Model file for the job. Use its own axes, mm. A direction names the side the tool comes from. Round coordinates to 2 decimals unless told otherwise and drop trailing zeros. Order: outer loops, then holes, each group sorted by start corner. A loop starts at its lowest first (then second) coordinate and runs counter-clockwise, first axis right, second up. Notation, with made-up numbers: (20, 87) -> (50, 87) arc R25 cw to (50, 101) -> close; hole circle Ø6 at (-10.75, 57.5). An arc over 180 degrees is marked (long way). Put each result on its own line as item: value. Start each with the question number.
Q1. Cut at C-C, the plane x = 2. List the corners of the cut face in (y, z), and give its area (3 significant figures).
Q2. Probe L1, parallel to Z at x = 3.5, y = 2.5; L2, parallel to Y at x = 9.62, z = 1.5; L3, parallel to X at y = -2, z = -49. List the from-to ranges inside material, lowest first.
Q3. 3-axis set-ups, long thin cutter, end or side, ignore diameter. For faces 4 (the face through (-15.889, 10.106, -54.845)), 5 (the face through (-11.96, 18.73, -4.93)), 6 (the face through (-13, 0.05, -4)), 7 (the face through (9.322, 1.373, 1.217)): which of +Z, -Z, +X, -X, +Y, -Y reach the whole face in a straight line?
Q4. Flat gauge pins, fed straight in: P1, Ø6, axis at x = -12.5, z = -17.5, coming from the -Y side; P2, Ø3, axis at x = -14.5, z = -6.5, coming from the -Y side; P3, Ø2, axis at x = 9.62, y = 2.715, coming from the +Z side; P4, Ø8, axis at x = -13, z = -5.5, coming from the +Y side. Where does each tip first touch, or does it go through?
Q5. Cut at D-D, the plane x = 9.62. List the corners of the cut face in (y, z) (3 decimals), and give its area (3 significant figures).
Q6. Cut at B-B, the plane y = 10. List the corners of the cut face in (x, z) (3 decimals).
Q7. Pull direction Y, two halves, no side cores. Call faces 1 (the face through (16.726, 11.363, 1.217)), 2 (the face through (-13, 0.05, -52)), 3 (the face through (-17.889, 10.245, -57.245)): released by +Y, released by -Y, zero draft, split by the parting line, or undercut.
Q8. Cut at A-A, the plane z = -8.5. List the corners of the cut face in (x, y), and give its area (3 significant figures).
from build123d import *

# Parameters (mm, degrees)
BOSS_EXTRUDE1_DEPTH = 2.4
BOSS_EXTRUDE2_DEPTH = 2.4
SKETCH2_W           = 2
SKETCH2_H           = 35
BOSS_EXTRUDE3_DEPTH = 60.848228
CUT_EXTRUDE1_REACH  = 62.848
SKETCH4_R           = 1.575
CUT_EXTRUDE2_REACH  = 62.848
SKETCH6_R           = 3.41
SKETCH6_R_2         = 1.375
FILLET1_R           = 4
BOSS_EXTRUDE4_DEPTH = 1.2
BOSS_EXTRUDE5_DEPTH = 1.2


with BuildPart() as part:
    # Sketch1 → Boss-Extrude1 (new body)
    with BuildSketch(Plane.XY):
        with BuildLine():
            Line((12.127473017, -0.607666052), (-17.03, -7.5))
            Line((-17.03, -7.5), (-17.03, 27.5))
            Line((-17.03, 27.5), (12.127473017, 20.607666052))
            ThreePointArc((12.127473017, 20.607666052), (20.52, 10), (12.127473017, -0.607666052))
        make_face()
    extrude(amount=BOSS_EXTRUDE1_DEPTH)



with BuildPart() as body_2:
    # Sketch3 → Boss-Extrude2 (new body)
    with BuildSketch(Plane(origin=(0, 0, -56.04822809), x_dir=(-1, 0, 0), z_dir=(0, 0, -1))):
        with BuildLine():
            Line((-12.127473017, -0.607666052), (17.03, -7.5))
            Line((17.03, -7.5), (17.03, 27.5))
            Line((17.03, 27.5), (-12.127473017, 20.607666052))
            ThreePointArc((-12.127473017, 20.607666052), (-20.52, 10), (-12.127473017, -0.607666052))
        make_face()
    extrude(amount=BOSS_EXTRUDE2_DEPTH)


with BuildPart() as part_1:
    add(part.part)

    add(body_2.part)  # Boss-Extrude3 merges body 2
    # Sketch2 → Boss-Extrude3 (add)
    with BuildSketch(Plane.XY.offset(2.4)):
        with Locations((-18.03, 10)):
            Rectangle(SKETCH2_W, SKETCH2_H)
    extrude(amount=-BOSS_EXTRUDE3_DEPTH)

    # Sketch4 → Cut-Extrude1 (cut, up to next)
    with BuildSketch(Plane(origin=(0, 0, -58.44822809), x_dir=(-1, 0, 0), z_dir=(0, 0, -1)), mode=Mode.PRIVATE) as cut_extrude1_sk1:
        with Locations((-9.62, 10)):
            Circle(SKETCH4_R)
    cut_extrude1_tool1 = extrude(cut_extrude1_sk1.sketch, amount=-CUT_EXTRUDE1_REACH, mode=Mode.PRIVATE) & part_1.part
    add(cut_extrude1_tool1.solids().sort_by_distance((9.62, 10, -58.448228))[0], mode=Mode.SUBTRACT)

    # Sketch6 → Cut-Extrude2 (cut, up to next)
    with BuildSketch(Plane.XY.offset(2.4), mode=Mode.PRIVATE) as cut_extrude2_sk1:
        with Locations((9.62, 10)):
            Circle(SKETCH6_R)
    cut_extrude2_tool1 = extrude(cut_extrude2_sk1.sketch, amount=-CUT_EXTRUDE2_REACH, mode=Mode.PRIVATE) & part_1.part
    add(cut_extrude2_tool1.solids().sort_by_distance((9.62, 10, 2.4))[0], mode=Mode.SUBTRACT)
    # Sketch6 → Cut-Extrude2 (cut, up to next)
    with BuildSketch(Plane.XY.offset(2.4), mode=Mode.PRIVATE) as cut_extrude2_sk2:
        with Locations((2.335, 10)):
            Circle(SKETCH6_R_2)
    cut_extrude2_tool2 = extrude(cut_extrude2_sk2.sketch, amount=-CUT_EXTRUDE2_REACH, mode=Mode.PRIVATE) & part_1.part
    add(cut_extrude2_tool2.solids().sort_by_distance((2.335, 10, 2.4))[0], mode=Mode.SUBTRACT)
    # Sketch6 → Cut-Extrude2 (cut, up to next)
    with BuildSketch(Plane.XY.offset(2.4), mode=Mode.PRIVATE) as cut_extrude2_sk3:
        with Locations((9.62, 17.285)):
            Circle(SKETCH6_R_2)
    cut_extrude2_tool3 = extrude(cut_extrude2_sk3.sketch, amount=-CUT_EXTRUDE2_REACH, mode=Mode.PRIVATE) & part_1.part
    add(cut_extrude2_tool3.solids().sort_by_distance((9.62, 17.285, 2.4))[0], mode=Mode.SUBTRACT)
    # Sketch6 → Cut-Extrude2 (cut, up to next)
    with BuildSketch(Plane.XY.offset(2.4), mode=Mode.PRIVATE) as cut_extrude2_sk4:
        with Locations((16.905, 10)):
            Circle(SKETCH6_R_2)
    cut_extrude2_tool4 = extrude(cut_extrude2_sk4.sketch, amount=-CUT_EXTRUDE2_REACH, mode=Mode.PRIVATE) & part_1.part
    add(cut_extrude2_tool4.solids().sort_by_distance((16.905, 10, 2.4))[0], mode=Mode.SUBTRACT)
    # Sketch6 → Cut-Extrude2 (cut, up to next)
    with BuildSketch(Plane.XY.offset(2.4), mode=Mode.PRIVATE) as cut_extrude2_sk5:
        with Locations((9.62, 2.715)):
            Circle(SKETCH6_R_2)
    cut_extrude2_tool5 = extrude(cut_extrude2_sk5.sketch, amount=-CUT_EXTRUDE2_REACH, mode=Mode.PRIVATE) & part_1.part
    add(cut_extrude2_tool5.solids().sort_by_distance((9.62, 2.715, 2.4))[0], mode=Mode.SUBTRACT)

    # Fillet1
    fillet1_edges = [part_1.edges().sort_by_distance(p)[0] for p in [
        (-19.03, 10, -58.448228),
        (-19.03, 10, 2.4),
        (-17.03, 10, 0),
        (-17.03, 10, -56.04822809),
    ]]
    fillet(fillet1_edges, radius=FILLET1_R)

    # Sketch9 → Boss-Extrude4 (add, symmetric)
    with BuildSketch(Plane(origin=(0, 18.75, 0), x_dir=(-1, 0, 0), z_dir=(0, -1, 0))):
        Polygon((17.03, 46.04822809), (7.03, 56.04822809), (17.03, 56.04822809), align=None)
        Polygon((17.03, 10), (17.03, 0), (7.03, 0), align=None)
    extrude(amount=BOSS_EXTRUDE4_DEPTH, both=True)

    # Sketch10 → Boss-Extrude5 (add, symmetric)
    with BuildSketch(Plane(origin=(0, 1.25, 0), x_dir=(-1, 0, 0), z_dir=(0, -1, 0))):
        Polygon((7.03, 56.04822809), (17.03, 56.04822809), (17.03, 46.04822809), align=None)
        Polygon((17.03, 10), (17.03, 0), (7.03, 0), align=None)
    extrude(amount=BOSS_EXTRUDE5_DEPTH, both=True)


solid = part_1.part
Ans:
1. outline: (-3, -58.45) -> (23, -58.45) -> (23, -56.05) -> (-3, -56.05) -> close; (-3, 0) -> (8.67, 0) -> (8.67, 2.4) -> (-3, 2.4) -> close; (11.33, 0) -> (23, 0) -> (23, 2.4) -> (11.33, 2.4) -> close
1. area: 118 mm^2
2. L1: z = -58.45 to -56.05, 0 to 2.4
2. L2: y = -1.2 to 1.34, 4.09 to 6.59, 13.41 to 15.91, 18.66 to 21.2
2. L3: x = -19.03 to -17.03
3. face 4: +X
3. face 5: +X, +Y, -Y
3. face 6: +X, -Y
3. face 7: +Z
4. P1: passes through
4. P2: stops at y = 0.05
4. P3: stops at z = -56.05
4. P4: stops at y = 19.95
5. outline: (-1.2, -58.448) -> (8.425, -58.448) -> (8.425, -56.048) -> (-1.2, -56.048) -> close; (-1.2, 0) -> (1.34, 0) -> (1.34, 2.4) -> (-1.2, 2.4) -> close; (4.09, 0) -> (6.59, 0) -> (6.59, 2.4) -> (4.09, 2.4) -> close; (11.575, -58.448) -> (21.2, -58.448) -> (21.2, -56.048) -> (11.575, -56.048) -> close; (13.41, 0) -> (15.91, 0) -> (15.91, 2.4) -> (13.41, 2.4) -> close; (18.66, 0) -> (21.2, 0) -> (21.2, 2.4) -> (18.66, 2.4) -> close
5. area: 70.4 mm^2
6. outline: (-19.03, -54.448) arc R4 ccw to (-15.03, -58.448) -> (8.045, -58.448) -> (8.045, -56.048) -> (-13.03, -56.048) arc R4 cw to (-17.03, -52.048) -> (-17.03, -4) arc R4 cw to (-13.03, 0) -> (0.96, 0) -> (0.96, 2.4) -> (-15.03, 2.4) arc R4 ccw to (-19.03, -1.6) -> close; (3.71, 0) -> (6.21, 0) -> (6.21, 2.4) -> (3.71, 2.4) -> close; (11.195, -58.448) -> (20.52, -58.448) -> (20.52, -56.048) -> (11.195, -56.048) -> close; (13.03, 0) -> (15.53, 0) -> (15.53, 2.4) -> (13.03, 2.4) -> close; (18.28, 0) -> (20.52, 0) -> (20.52, 2.4) -> (18.28, 2.4) -> close
7. face 1: undercut
7. face 2: released by -Y
7. face 3: zero draft
8. outline: (-19.03, -7.5) -> (-17.03, -7.5) -> (-17.03, 0.05) -> (-15.53, 0.05) -> (-15.53, 2.45) -> (-17.03, 2.45) -> (-17.03, 17.55) -> (-15.53, 17.55) -> (-15.53, 19.95) -> (-17.03, 19.95) -> (-17.03, 27.5) -> (-19.03, 27.5) -> close
8. area: 77.2 mm^2
